```python
from build123d import *

# Parameters (mm, degrees)
EXTRUDE_THIN1_DEPTH = 50
CHAMFER1_SIZE       = 5
SKETCH2_R           = 11
SKETCH2_R_2         = 1.5
CUT_EXTRUDE1_DEPTH  = 10


with BuildPart() as part:
    # Sketch1 → Extrude-Thin1 (new body)
    with BuildSketch(Plane.XY):
        Polygon((52, 0), (0, 0), (0, 52), (-2, 52), (-2, -2), (52, -2), align=None)
    extrude(amount=EXTRUDE_THIN1_DEPTH)

    # Chamfer1
    chamfer1_edges = [part.edges().sort_by_distance(p)[0] for p in [
        (-1, 52, 50),
        (-1, 52, 0),
        (52, -1, 0),
        (52, -1, 50),
    ]]
    chamfer(chamfer1_edges, length=CHAMFER1_SIZE)

    # Sketch2 → Cut-Extrude1 (cut)
    with BuildSketch(Plane.XZ.offset(2)):
        with Locations((31, 25)):
            Circle(SKETCH2_R)
        with Locations((15.5, 40.5)):
            Circle(SKETCH2_R_2)
        with Locations((46.5, 40.5)):
            Circle(SKETCH2_R_2)
        with Locations((46.5, 9.5)):
            Circle(SKETCH2_R_2)
        with Locations((15.5, 9.5)):
            Circle(SKETCH2_R_2)
    extrude(amount=-CUT_EXTRUDE1_DEPTH, mode=Mode.SUBTRACT)


solid = part.part
```
Model file for the job. Use its own axes, mm. A direction names the side the tool comes from. Give positions to 0.01 mm unless a question says otherwise; leave off trailing zeros. Loops run counter-clockwise (first coordinate to the right, second up) from the corner with the lowest first, then second, coordinate; pieces in that order, holes last. Notation, with made-up numbers: (27.5, 45.25) - (33.5, 45.25) arc R26 cw to (33.5, 71.25) - close; hole circle Ø1 at (-36, -6.5). An arc over 180 degrees is marked (long way). One line per item, written item: value. Start each with the question number.
1. Pull direction X, two halves, no side cores. Call faces 3 (the flat face through (49, -1, 2)), 4 (the cylindrical face through (45.3, -1, 39.6)), 5 (the flat face through (-1, 49, 2)): pulls with the +X half, pulls with the -X half, needs draft (parallel to the pull), parting line crosses it, or undercut.
2. Probe L1, parallel to Z at x = 46.5, y = -1.05; L2, parallel to Z at x = 31, y = -1.3; L3, parallel to Z at x = 15, y = -1. List the from-to ranges inside material, lowest first. Write a range as from..to.
3. Slice it at D-D (x = 31). List the corners of the cut face in (y, z), plus the area to 3 significant figures.
4. Slice it at C-C (z = 40.5). List the corners of the cut face in (x, y), plus the area to 3 significant figures.
5. Slice it at A-A (z = 25). List the corners of the cut face in (x, y), plus the area to 3 significant figures.
6. Slice it at B-B (x = 15.5). List the corners of the cut face in (y, z).
7. Which spindle directions (+Z, -Z, +X, -X, +Y, -Y) get a long thin tool onto all of the face, cutting with end or side? Do faces 1 (the flat face through (-1, 52, 25)), 2 (the flat face through (0, 26, 25)). Say none if no direction does.
8. Pin check, flat tips, straight feed: pin 1 (1.8 mm diameter, centred on x = 15.5, z = 40.5, fed in from -Y); pin 2 (1.5 mm diameter, centred on y = 4.5, z = 6.5, fed in from +X); pin 3 (5 mm diameter, centred on x = 46.5, z = 9.5, fed in from +Y). Stop position of each tip, or through.
Solution:
1. face 3: pulls with the +X half
1. face 4: undercut
1. face 5: needs draft
2. L1: z = 0..8, 11..39, 42..50
2. L2: z = 0..14, 36..50
2. L3: z = 0..8.09, 10.91..39.09, 41.91..50
3. outline: (-2, 0) - (0, 0) - (0, 14) - (-2, 14) - close; (-2, 36) - (0, 36) - (0, 50) - (-2, 50) - close
3. area: 56.0 mm^2
4. outline: (-2, -2) - (14, -2) - (14, 0) - (0, 0) - (0, 52) - (-2, 52) - close; (17, -2) - (45, -2) - (45, 0) - (17, 0) - close; (48, -2) - (52, -2) - (52, 0) - (48, 0) - close
4. area: 200 mm^2
5. outline: (-2, -2) - (20, -2) - (20, 0) - (0, 0) - (0, 52) - (-2, 52) - close; (42, -2) - (52, -2) - (52, 0) - (42, 0) - close
5. area: 168 mm^2
6. outline: (-2, 0) - (0, 0) - (0, 8) - (-2, 8) - close; (-2, 11) - (0, 11) - (0, 39) - (-2, 39) - close; (-2, 42) - (0, 42) - (0, 50) - (-2, 50) - close
7. face 1: +Z, -Z, +X, -X, +Y
7. face 2: +Z, -Z, +X, +Y
8. pin 1: passes through
8. pin 2: stops at x = 0
8. pin 3: stops at y = 0
